from build123d import *

# Parameters (mm, degrees)
SALIENTE_EXTRUIR1_DEPTH = 30
CROQUIS2_W              = 26
CROQUIS2_H              = 16
CORTAR_EXTRUIR1_DEPTH   = 51
CROQUIS3_W              = 26
CROQUIS3_H              = 12
CORTAR_EXTRUIR2_DEPTH   = 31
CORTAR_EXTRUIR4_DEPTH   = 31
CORTAR_EXTRUIR5_DEPTH   = 31
CORTAR_EXTRUIR6_DEPTH   = 31


with BuildPart() as part:
    # Croquis1 → Saliente-Extruir1 (new body, symmetric)
    with BuildSketch(Plane.XY):
        Polygon((0, 0), (50, 0), (50, 57), (30, 57), (30, 100), (0, 100), align=None)
    extrude(amount=SALIENTE_EXTRUIR1_DEPTH, both=True)

    # Croquis2 → Cortar-Extruir1 (cut, through all)
    with BuildSketch(Plane(origin=(50, 0, 0), x_dir=(0, 0, -1), z_dir=(1, 0, 0))):
        with Locations((-14, 48)):
            Rectangle(CROQUIS2_W, CROQUIS2_H)
        with Locations((14, 48)):
            Rectangle(CROQUIS2_W, CROQUIS2_H)
        with Locations((-14, 30)):
            Rectangle(CROQUIS2_W, CROQUIS2_H)
        with Locations((14, 30)):
            Rectangle(CROQUIS2_W, CROQUIS2_H)
        with Locations((-14, 12)):
            Rectangle(CROQUIS2_W, CROQUIS2_H)
        with Locations((14, 12)):
            Rectangle(CROQUIS2_W, CROQUIS2_H)
    extrude(amount=-CORTAR_EXTRUIR1_DEPTH, mode=Mode.SUBTRACT)

    # Croquis3 → Cortar-Extruir2 (cut, through all)
    with BuildSketch(Plane(origin=(30, 0, 0), x_dir=(0, 0, -1), z_dir=(1, 0, 0))):
        with Locations((-14, 92)):
            Rectangle(CROQUIS3_W, CROQUIS3_H)
        with Locations((14, 92)):
            Rectangle(CROQUIS3_W, CROQUIS3_H)
    extrude(amount=-CORTAR_EXTRUIR2_DEPTH, mode=Mode.SUBTRACT)

    # Croquis4 → Cortar-Extruir4 (cut, through all)
    with BuildSketch(Plane(origin=(30, 0, 0), x_dir=(0, 0, -1), z_dir=(1, 0, 0))):
        Polygon((-23.506160606, 60.828952145), (-22.677208461, 60), (-14.727245643, 60), (-14.116440614, 60.610805028), (-14.166440614, 60.660805028), (-14.216440614, 60.710805028), (-18.920374168, 65.414738582), align=None)
        Polygon((-12.920374168, 71.414738582), (-17.506160606, 66.828952145), (-12.702227052, 62.025018591), (-8.116440614, 66.610805028), align=None)
        Polygon((-6.876072053, 77.459040697), (-11.506160606, 72.828952145), (-6.702227052, 68.025018591), (-2.072138499, 72.655107144), align=None)
        Polygon((-0.831769938, 83.503342813), (-5.46185849, 78.87325426), (-0.657924937, 74.069320706), (3.972163616, 78.699409259), align=None)
        Polygon((1.5, 84), (5.386377179, 80.113622821), (9.272754357, 84), align=None)
        Polygon((-14.159291936, 84), (-22.677208461, 84), (-18.418250198, 79.741041737), align=None)
        Polygon((-10.588604231, 84), (-6.876072053, 80.287467822), (-3.163539875, 84), align=None)
        Polygon((-17.004036636, 78.326828175), (-12.920374168, 74.243165707), (-8.290285615, 78.87325426), (-12.373948083, 82.956916728), align=None)
        Polygon((-23.004036636, 72.326828175), (-18.920374168, 68.243165707), (-14.33458773, 72.828952145), (-18.418250198, 76.912614613), align=None)
        Polygon((-27, 64.322791539), (-24.920374168, 62.243165707), (-20.33458773, 66.828952145), (-24.418250198, 70.912614613), (-27, 68.330864811), align=None)
        Polygon((-27, 61.494364414), (-27, 60.263539875), (-27, 60.163539875), (-26.33458773, 60.828952145), align=None)
        Polygon((27, 67.760177106), (23.866973526, 70.89320358), (19.236884973, 66.263115027), (24.040818527, 61.459181473), (27, 64.418362946), align=None)
        Polygon((13.588604231, 84), (17.64882641, 79.939777821), (21.709048589, 84), align=None)
        Polygon((11.430679294, 83.329497812), (6.800590741, 78.699409259), (11.604524295, 73.895475705), (16.234612848, 78.525564258), align=None)
        Polygon((5.386377179, 77.285195697), (0.756288626, 72.655107144), (5.560222179, 67.85117359), (10.190310732, 72.481262143), align=None)
        Polygon((-0.657924937, 71.240893581), (-5.28801349, 66.610805028), (-0.484079936, 61.806871475), (4.146008617, 66.436960028), align=None)
        Polygon((-1.948293498, 60.442657912), (-1.998293498, 60.492657912), (-6.702227052, 65.196591466), (-11.28801349, 60.610805028), (-10.677208461, 60), (-2.290951411, 60), (-1.898293498, 60.392657912), align=None)
        Polygon((27, 79.848781336), (23.693128525, 83.155652811), (19.063039972, 78.525564258), (23.866973526, 73.721630704), (27, 76.854657178), align=None)
        Polygon((10.364155733, 60.218812911), (10.314155733, 60.268812911), (5.560222179, 65.022746465), (0.930133627, 60.392657912), (1.322791539, 60), (10.145342822, 60), align=None)
        Polygon((17.64882641, 77.111350696), (13.018737857, 72.481262143), (17.822671411, 67.677328589), (22.452759964, 72.307417142), align=None)
        Polygon((11.604524295, 71.067048581), (6.974435742, 66.436960028), (11.778369296, 61.633026474), (16.408457848, 66.263115027), align=None)
        Polygon((-27, 79.326616872), (-27, 76.322791539), (-24.418250198, 73.741041737), (-19.832463761, 78.326828175), (-23.916126229, 82.410490643), align=None)
        Polygon((22.581637054, 60), (22.626604965, 60.044967911), (17.822671411, 64.848901464), (13.192582858, 60.218812911), (13.411395769, 60), align=None)
        Polygon((-27, 71.159291936), (-25.832463761, 72.326828175), (-27, 73.494364414), align=None)
        Polygon((27, 74.026230054), (25.281187089, 72.307417142), (27, 70.588604231), align=None)
        Polygon((27, 61.589935821), (25.455032089, 60.044967911), (25.5, 60), (27, 60), align=None)
    extrude(amount=-CORTAR_EXTRUIR4_DEPTH, mode=Mode.SUBTRACT)

    # Croquis5 → Cortar-Extruir5 (cut, through all)
    with BuildSketch(Plane(origin=(30, 0, 0), x_dir=(0, 0, -1), z_dir=(1, 0, 0))):
        Polygon((-27.085333176, 82.379183427), (-27.085333176, 84.183862587), (-25.280654015, 84.183862587), align=None)
    extrude(amount=-CORTAR_EXTRUIR5_DEPTH, mode=Mode.SUBTRACT)

    # Croquis6 → Cortar-Extruir6 (cut, through all)
    with BuildSketch(Plane(origin=(30, 0, 0), x_dir=(0, 0, -1), z_dir=(1, 0, 0))):
        Polygon((27.009208932, 83.908640009), (27.009208932, 81.911495936), (25.012064859, 83.908640009), align=None)
    extrude(amount=-CORTAR_EXTRUIR6_DEPTH, mode=Mode.SUBTRACT)


solid = part.part
Geometry check sheet. Reference: the model listing, model coordinates, mm. Give positions to 0.01 mm unless a question says otherwise; leave off trailing zeros. Order: outer loops, then holes, each group sorted by start corner. A loop starts at its lowest first (then second) coordinate and runs counter-clockwise, first axis right, second up.
1. Depth check by flat-ended pin: pin 1 (1.5 mm diameter, centred on y = 64.5, z = 20, fed in from +X); pin 2 (8 mm diameter, centred on x = 36, z = 16.5, fed in from +Y). Enter the tip coordinate at first touch or a pass-through.
Completed:
pin 1: stops at x = 30
pin 2: stops at y = 57
2. Sectioned sample at C-C (y = 92). Record the boundary of the cut face in (x, z).
Completed:
outline: (0, -30) - (30, -30) - (30, -27) - (0, -27) - close; (0, -1) - (30, -1) - (30, 1) - (0, 1) - close; (0, 27) - (30, 27) - (30, 30) - (0, 30) - close
3. Sectioned sample at B-B (x = 42). Record the boundary of the cut face in (y, z), then the cut area to 3 significant figures.
Completed:
outline: (0, -30) - (57, -30) - (57, 30) - (0, 30) - close; hole (4, -27) - (20, -27) - (20, -1) - (4, -1) - close; hole (4, 1) - (20, 1) - (20, 27) - (4, 27) - close; hole (22, -27) - (38, -27) - (38, -1) - (22, -1) - close; hole (22, 1) - (38, 1) - (38, 27) - (22, 27) - close; hole (40, -27) - (56, -27) - (56, -1) - (40, -1) - close; hole (40, 1) - (56, 1) - (56, 27) - (40, 27) - close
area: 924 mm2
4. Sectioned sample at A-A (y = 24). Record the boundary of the cut face in (x, z), then the cut area to 3 significant figures.
Completed:
outline: (0, -30) - (50, -30) - (50, -27) - (0, -27) - close; (0, -1) - (50, -1) - (50, 1) - (0, 1) - close; (0, 27) - (50, 27) - (50, 30) - (0, 30) - close
area: 400 mm2
5. Draft check along Y on faces 1 (the face through (0, 62, 0)), 2 (the face through (40, 57, 0)), 3 (the face through (15.2, 63.9, -21.6)). Enter one of: pulls with the +Y half, pulls with the -Y half, needs draft (parallel to the pull), parting line crosses it, or undercut.
Completed:
face 1: needs draft
face 2: pulls with the +Y half
face 3: undercut
6. Sectioned sample at D-D (x = 27). State how many separate pieces and enclosed holes the cut face has, then the cut area to 3 significant figures.
Completed:
separate pieces: 1
enclosed holes: 36
area: 2,120 mm2
7. Scan lines: line 1 (Y direction, x = 42, z = 16.5); line 2 (Z direction, x = 38.5, y = 37); line 3 (X direction, y = 85, z = -9.5). Record each from-to range of solid material in increasing order.
Completed:
line 1: y = 0 to 4, 20 to 22, 38 to 40, 56 to 57
line 2: z = -30 to -27, -1 to 1, 27 to 30
line 3: x = 0 to 30
